from build123d import *

# Parameters (mm, degrees)
SKETCH1_W           = 265.950423439
SKETCH1_H           = 258.221174697
BASE_DEPTH          = 6
SKETCH2_W           = 6.892214754
SKETCH2_H           = 258.221174697
BOSS_EXTRUDE2_DEPTH = 80
FILLET1_R           = 5


with BuildPart() as part:
    # Sketch1 → Base (new body)
    with BuildSketch(Plane(origin=(0, 0, 0), x_dir=(1, 0, 0), z_dir=(0, 1, 0))):
        with Locations((-129.157291203, -107.886320424)):
            Rectangle(SKETCH1_W, SKETCH1_H)
    extrude(amount=BASE_DEPTH)

    # Sketch2 → Boss-Extrude2 (add)
    with BuildSketch(Plane(origin=(0, 6, 0), x_dir=(1, 0, 0), z_dir=(0, 1, 0))):
        with Locations((-258.686395546, -107.886320424)):
            Rectangle(SKETCH2_W, SKETCH2_H)
    extrude(amount=BOSS_EXTRUDE2_DEPTH)

    # Fillet1
    fillet1_edges = [part.edges().sort_by_distance(p)[0] for p in [
        (-255.240288169, 6, 107.886320423),
    ]]
    fillet(fillet1_edges, radius=FILLET1_R)


solid = part.part
Here's how the part is built. I have some questions about the finished solid (model axes, mm). A direction names the side the tool comes from. Coordinates: 2 decimals unless noted, no trailing zeros. Write each loop counter-clockwise with the first axis right and the second up, starting at its lowest first coordinate (ties: lowest second). Pieces come first, ordered by that corner, then holes.
Item 1: I want a section at C-C on x = -212.5. Write out the boundary of the cut face in (y, z), and give its area (3 significant figures).
Item 2: On a 3-axis mill with a long thin cutter (end or side, diameter ignored), from which of +Z, -Z, +X, -X, +Y, -Y can I reach the whole of each face in a straight line? I mean faces 1 (the flat face through (-125, 6, 106)), 2 (the flat face through (-259, 86, 106)). Say none if no direction works.
Item 3: I want a section at B-B on y = 42. Write out the boundary of the cut face in (x, z).
Item 4: Will these pins go through, and if not, where does the flat tip stop? pin 1 (1 mm diameter, centred on x = -53.5, z = 33, fed in from +Y); pin 2 (8 mm diameter, centred on y = 11.5, z = 202, fed in from +X); pin 3 (1 mm diameter, centred on y = 51.5, z = 144.5, fed in from +X).
Item 5: If I drill on line 1 (X direction, y = 36.5, z = 65); line 2 (Y direction, x = -75.5, z = 113); line 3 (X direction, y = 8, z = 91), over which ranges is the centre line in solid material (lowest first)?
Item 6: I want a section at A-A on z = 152.5. Write out the boundary of the cut face in (x, y).
Findings below:
1. outline: (0, -21.22) - (6, -21.22) - (6, 237) - (0, 237) - close
1. area: 1,550 mm2
2. face 1: +Z, -Z, +X, +Y
2. face 2: +Z, -Z, +X, -X, +Y
3. outline: (-262.13, -21.22) - (-255.24, -21.22) - (-255.24, 237) - (-262.13, 237) - close
4. pin 1: stops at y = 6
4. pin 2: stops at x = -253.81
4. pin 3: stops at x = -255.24
5. line 1: x = -262.13 to -255.24
5. line 2: y = 0 to 6
5. line 3: x = -262.13 to -254.24
6. outline: (-262.13, 0) - (3.82, 0) - (3.82, 6) - (-250.24, 6) arc R5 cw to (-255.24, 11) - (-255.24, 86) - (-262.13, 86) - close
